The model under review builds one solid part; all positions refer to its coordinate system, in mm. Face numbers are marked on the shaded views. A direction names the side the tool comes from. Round coordinates to 2 decimals unless told otherwise and drop trailing zeros. Loops run counter-clockwise (first coordinate to the right, second up) from the corner with the lowest first, then second, coordinate; pieces in that order, holes last. Notation, with made-up numbers: (18.5, 12) -> (61.5, 12) arc R13 cw to (61.5, 24) -> close; hole circle Ø3 at (89, 52.25). An arc over 180 degrees is marked (long way). Use a Markdown table: item, result. Add a question column.
1) Mouldability with a two-part tool opening along Y and no side actions: class the marked faces 3, 4, 5 and 6 as released by +Y, released by -Y, zero draft, split by the parting line, or undercut.
2) Wall thickness on probe 1 along Y at (x, z) = (0, -1.1); probe 2 along Z at (x, y) = (11, 1.5); probe 3 along Y at (x, z) = (-13, 1): over which ranges is each line inside the solid? List them lowest first.
3) Consider section B-B on x = 15.5. Give the boundary of the cut face in (y, z), plus the area to 3 significant figures.
4) Consider section A-A on z = -2. Give the boundary of the cut face in (x, y), plus the area to 3 significant figures.
5) Insertion check: pin 1 (5 mm diameter, centred on y = -3.5, z = 16.5, fed in from -X); pin 2 (4 mm diameter, centred on y = 3.5, z = 4.5, fed in from +X); pin 3 (2 mm diameter, centred on x = -6.5, y = -11.5, fed in from -Z). Each pin has a flat end and moves straight along its axis. Give the tip position at first contact, or say it passes through.
6) For the marked faces 1 and 2, list the 3-axis set-ups (+Z, -Z, +X, -X, +Y, -Y) from which the entire face can be reached by the end or side of a thin tool; tool diameter is ignored.
7) Consider section D-D on z = 3.5. Give the boundary of the cut face in (x, y), plus the area to 3 significant figures.
8) Consider section C-C on y = 15. Give the boundary of the cut face in (x, z).
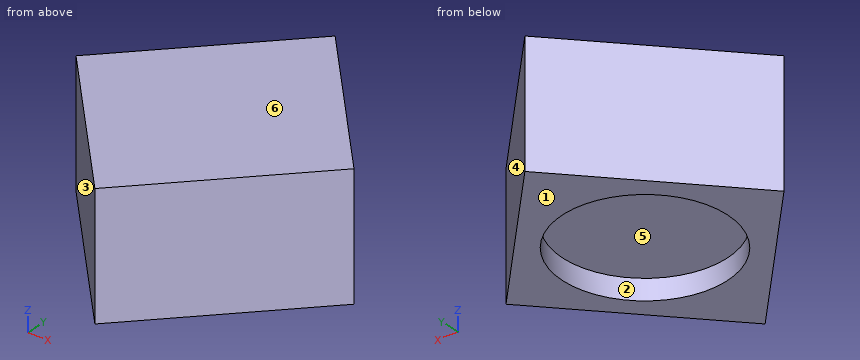
from build123d import *

# Parameters (mm, degrees)
F0_R      = 20
F1_DEPTH  = 25
F2_DEPTH  = 10
F3_DEPTH  = 15
F4_DEPTH  = 25
F5_DEPTH  = 5
F6_DEPTH  = 10
F7_DEPTH  = 10
F5_FACE_R = 20
F8_DEPTH  = 10


with BuildPart() as f1:
    # F0 (on Top) → F1 (new body)
    with BuildSketch(Plane.XY):
        Polygon((33.9652827231, 0), (0, 36.6927727154), (-33.9652827231, 0), (0, -36.6927727154), align=None)
        Circle(F0_R, mode=Mode.SUBTRACT)
    extrude(amount=F1_DEPTH)

    # F0 (on Top) → F2 (join)
    with BuildSketch(Plane.XY):
        Polygon((33.9652827231, 0), (0, 36.6927727154), (-33.9652827231, 0), (0, -36.6927727154), align=None)
        Circle(F0_R, mode=Mode.SUBTRACT)
    extrude(amount=F2_DEPTH)

    # F0 (on Top) → F3 (join)
    with BuildSketch(Plane.XY):
        Polygon((33.9652827231, 0), (0, 36.6927727154), (-33.9652827231, 0), (0, -36.6927727154), align=None)
        Circle(F0_R, mode=Mode.SUBTRACT)
        Circle(F0_R)
    extrude(amount=F3_DEPTH)

    # F0 (on Top) → F4 (join)
    with BuildSketch(Plane.XY):
        Circle(F0_R)
    extrude(amount=F4_DEPTH)

    # F0 (on Top) → F5 (join)
    with BuildSketch(Plane.XY):
        Polygon((33.9652827231, 0), (0, 36.6927727154), (-33.9652827231, 0), (0, -36.6927727154), align=None)
        Circle(F0_R, mode=Mode.SUBTRACT)
    extrude(amount=-F5_DEPTH)

    # F0 (on Top) → F6 (join)
    with BuildSketch(Plane.XY):
        Circle(F0_R)
    extrude(amount=F6_DEPTH)

    # F0 (on Top) → F7 (join)
    with BuildSketch(Plane.XY):
        Circle(F0_R)
    extrude(amount=F7_DEPTH)

    # F0 (on Top) + F5_face (on face) → F8 (join)
    with BuildSketch(Plane.XY):
        Circle(F0_R)
    with BuildSketch(Plane(origin=(0, 0, -5), x_dir=(1, 0, 0), z_dir=(0, 0, -1))):
        Polygon((0, 36.6927727154), (-33.9652827231, 0), (0, -36.6927727154), (33.9652827231, 0), align=None)
        Circle(F5_FACE_R, mode=Mode.SUBTRACT)
    extrude(amount=F8_DEPTH, dir=(0, 0, 1))


solid = f1.part
Result set:
| question | item | result |
|---|---|---|
| 1 | face 3 | released by -Y |
| 1 | face 4 | released by +Y |
| 1 | face 5 | undercut |
| 1 | face 6 | zero draft |
| 2 | probe 1 | -36.69 to -20, 20 to 36.69 |
| 2 | probe 2 | 0 to 25 |
| 2 | probe 3 | -22.65 to 22.65 |
| 3 | outline | (-19.95, -5) -> (-12.64, -5) -> (-12.64, 0) -> (12.64, 0) -> (12.64, -5) -> (19.95, -5) -> (19.95, 25) -> (-19.95, 25) -> close |
| 3 | area | 1,070 mm2 |
| 4 | outline | (-33.97, 0) -> (0, -36.69) -> (33.97, 0) -> (0, 36.69) -> close; hole circle Ø40 at (0, 0) |
| 4 | area | 1,240 mm2 |
| 5 | pin 1 | x = -33.04 |
| 5 | pin 2 | x = 32.58 |
| 5 | pin 3 | z = 0 |
| 6 | face 1 | -Z, +X, -X, +Y, -Y |
| 6 | face 2 | -Z |
| 7 | outline | (-33.97, 0) -> (0, -36.69) -> (33.97, 0) -> (0, 36.69) -> close |
| 7 | area | 2,490 mm2 |
| 8 | outline | (-20.08, -5) -> (-13.23, -5) -> (-13.23, 0) -> (13.23, 0) -> (13.23, -5) -> (20.08, -5) -> (20.08, 25) -> (-20.08, 25) -> close |
